Geometry: final body of the model. Coordinates: model frame, mm. A direction names the side the tool comes from. Round coordinates to 2 decimals unless told otherwise and drop trailing zeros. Loops run counter-clockwise (first coordinate to the right, second up) from the corner with the lowest first, then second, coordinate; pieces in that order, holes last. Notation, with made-up numbers: (-34, 3) - (-12, 3) arc R32 ccw to (-12, 31) - close; hole circle Ø2 at (16, 10). An arc over 180 degrees is marked (long way). Answer as a JSON object with one key per item and string values. Group by question number.
Item 1: Line query: line 1 (X direction, y = 3, z = 41); line 2 (Y direction, x = -20, z = 27.5); line 3 (Z direction, x = -6, y = 12). Output: solid intervals per line, ascending.
Item 2: Section A-A (y = 19). Return the cut outline in (x, z), plus the area to 3 significant figures.
Item 3: Section B-B (x = 8.5). Return the cut outline in (y, z).
Item 4: Draft query along X for faces 3 (the face through (22.45, -0.5, 35.72)), 4 (the face through (-22.5, 11.13, -0.45)), 5 (the face through (0, 11, 0)). Return one class per face: released by +X, released by -X, zero draft, split by the parting line, or undercut.
Item 5: Reachability of faces 1 (the face through (-22.45, -0.5, 34.78)), 2 (the face through (21.4, 0.57, 35.72)) from +Z, -Z, +X, -X, +Y, -Y: full face, straight path, thin tool, end or side. Return the list, or none.
Item 6: Section C-C (z = 7.5). Return the cut outline in (x, y).
Item 7: First-contact query: pin 1 (1.2 mm diameter, centred on y = -1, z = 35, fed in from +X); pin 2 (9 mm diameter, centred on x = 6.5, y = 12, fed in from +Z); pin 3 (0.8 mm diameter, centred on y = -0.5, z = 39, fed in from -X). Flat tips, straight axial feed; report the tip coordinate or a pass-through.
Item 8: Section D-D (z = 64.5). Return the cut outline in (x, y), plus the area to 3 significant figures.
```python
from build123d import *

# Parameters (mm, degrees)
BOX002_W     = 36
BOX002_H     = 20.5
BOX002_DEPTH = 70
FILLET004_R  = 6
BOX_W        = 44
BOX_H        = 22
BOX_DEPTH    = 70
FILLET_R     = 2
FILLET005_R  = 2
BOX003_W     = 47
BOX003_H     = 25
BOX003_DEPTH = 70
FILLET006_R  = 3.5
FILLET007_R  = 3.5


with BuildPart() as fillet004:
    # Box002 → Box002 (new body)
    with BuildSketch(Plane(origin=(-18, -10, 4), x_dir=(1, 0, 0), z_dir=(0, 0, 1))):
        with Locations((18, 10.25)):
            Rectangle(BOX002_W, BOX002_H)
    extrude(amount=BOX002_DEPTH)

    # Fillet004
    fillet004_edges = [fillet004.edges().sort_by_distance(p)[0] for p in [
        (-18, 0.25, 4),
        (18, 0.25, 4),
    ]]
    fillet(fillet004_edges, radius=FILLET004_R)


with BuildPart() as fusion:
    # Box → Box (new body)
    with BuildSketch(Plane(origin=(-22, 0, 0), x_dir=(1, 0, 0), z_dir=(0, 0, 1))):
        with Locations((22, 11)):
            Rectangle(BOX_W, BOX_H)
    extrude(amount=BOX_DEPTH)

    # Fillet
    fillet_edges = [fusion.edges().sort_by_distance(p)[0] for p in [
        (-22, 11, 0),
        (22, 11, 0),
    ]]
    fillet(fillet_edges, radius=FILLET_R)

    # Fillet005
    fillet005_edges = [fusion.edges().sort_by_distance(p)[0] for p in [
        (22, 0, 36),
        (22, 22, 36),
    ]]
    fillet(fillet005_edges, radius=FILLET005_R)

    # Fusion: union Fillet004
    add(fillet004.part)


with BuildPart() as cut:
    # Box003 → Box003 (new body)
    with BuildSketch(Plane(origin=(-23.5, -1.5, -1.5), x_dir=(1, 0, 0), z_dir=(0, 0, 1))):
        with Locations((23.5, 12.5)):
            Rectangle(BOX003_W, BOX003_H)
    extrude(amount=BOX003_DEPTH)

    # Fillet006
    fillet006_edges = [cut.edges().sort_by_distance(p)[0] for p in [
        (-23.5, 11, -1.5),
        (23.5, 11, -1.5),
    ]]
    fillet(fillet006_edges, radius=FILLET006_R)

    # Fillet007
    fillet007_edges = [cut.edges().sort_by_distance(p)[0] for p in [
        (0, -1.5, -1.5),
        (0, 23.5, -1.5),
    ]]
    fillet(fillet007_edges, radius=FILLET007_R)

    # Cut: cut Fusion
    add(fusion.part, mode=Mode.SUBTRACT)


solid = cut.part
```
Values:
{
 "1": {"line 1": "x = -23.5 to -22, 22 to 23.5", "line 2": "y = -1.5 to 0, 22 to 23.5", "line 3": "z = -1.5 to 0"},
 "2": {"outline": "(-23.5, 2) arc R3.5 ccw to (-20, -1.5) - (20, -1.5) arc R3.5 ccw to (23.5, 2) - (23.5, 68.5) - (22, 68.5) - (22, 2) arc R2 cw to (20, 0) - (-20, 0) arc R2 cw to (-22, 2) - (-22, 68.5) - (-23.5, 68.5) - close", "area": "272 mm^2"},
 "3": {"outline": "(-1.5, 2) arc R3.5 ccw to (2, -1.5) - (20, -1.5) arc R3.5 ccw to (23.5, 2) - (23.5, 68.5) - (22, 68.5) - (22, 2) arc R2 cw to (20, 0) - (2, 0) arc R2 cw to (0, 2) - (0, 4) - (-1.5, 4) - close"},
 "4": {"face 3": "released by +X", "face 4": "released by -X", "face 5": "undercut"},
 "5": {"face 1": "+Z, -Z, -X, -Y", "face 2": "+Z"},
 "6": {"outline": "(-23.5, 2) arc R3.5 ccw to (-20, -1.5) - (-17.45, -1.5) - (-17.45, 0) - (-20, 0) arc R2 cw to (-22, 2) - (-22, 20) arc R2 cw to (-20, 22) - (20, 22) arc R2 cw to (22, 20) - (22, 2) arc R2 cw to (20, 0) - (17.45, 0) - (17.45, -1.5) - (20, -1.5) arc R3.5 ccw to (23.5, 2) - (23.5, 20) arc R3.5 ccw to (20, 23.5) - (-20, 23.5) arc R3.5 ccw to (-23.5, 20) - close"},
 "7": {"pin 1": "stops at x = 22.55", "pin 2": "stops at z = 0", "pin 3": "stops at x = -22.8"},
 "8": {"outline": "(-23.5, 2) arc R3.5 ccw to (-20, -1.5) - (-18, -1.5) - (-18, 0) - (-20, 0) arc R2 cw to (-22, 2) - (-22, 20) arc R2 cw to (-20, 22) - (20, 22) arc R2 cw to (22, 20) - (22, 2) arc R2 cw to (20, 0) - (18, 0) - (18, -1.5) - (20, -1.5) arc R3.5 ccw to (23.5, 2) - (23.5, 20) arc R3.5 ccw to (20, 23.5) - (-20, 23.5) arc R3.5 ccw to (-23.5, 20) - close", "area": "146 mm^2"}
}
